Design review of the part built by this model. Coordinates are the model's own, in mm. Round coordinates to 2 decimals unless told otherwise and drop trailing zeros. Loops run counter-clockwise (first coordinate to the right, second up) from the corner with the lowest first, then second, coordinate; pieces in that order, holes last. Notation, with made-up numbers: (2.25, 9) - (48.25, 9) arc R21 ccw to (48.25, 27) - close; hole circle Ø5 at (-12.75, 34.5). An arc over 180 degrees is marked (long way). Return JSON: item names as keys, results as strings. Group by question number.
from build123d import *

# Parameters (mm, degrees)
SKETCH1_W           = 144.4
SKETCH1_H           = 144.4
BOSS_EXTRUDE1_DEPTH = 3
SKETCH2_W           = 20.628571
SKETCH2_H           = 3
SKETCH2_W_2         = 3
SKETCH2_H_2         = 19.771429
SKETCH2_H_3         = 19.83347722
SKETCH2_H_4         = 19.833479362
SKETCH2_H_5         = 19.771431142
CUT_EXTRUDE1_DEPTH  = 4
SKETCH3_R           = 1
CUT_EXTRUDE2_DEPTH  = 4
SKETCH4_R           = 4.8
CUT_EXTRUDE3_DEPTH  = 4


with BuildPart() as part:
    # Sketch1 → Boss-Extrude1 (new body)
    with BuildSketch(Plane.XY):
        Rectangle(SKETCH1_W, SKETCH1_H)
    extrude(amount=BOSS_EXTRUDE1_DEPTH)

    # Sketch2 → Cut-Extrude1 (cut, through all)
    with BuildSketch(Plane(origin=(0, 0, 0), x_dir=(-1, 0, 0), z_dir=(0, 0, -1))):
        with Locations((-41.257140929, 70.7)):
            Rectangle(SKETCH2_W, SKETCH2_H)
        with Locations((1.071e-06, 70.7)):
            Rectangle(SKETCH2_W, SKETCH2_H)
        with Locations((41.257143071, 70.7)):
            Rectangle(SKETCH2_W, SKETCH2_H)
        with Locations((70.7, 39.542856929)):
            Rectangle(SKETCH2_W_2, SKETCH2_H_2)
        with Locations((70.7, -1.071e-06)):
            Rectangle(SKETCH2_W_2, SKETCH2_H_2)
        with Locations((70.7, -39.573883181)):
            Rectangle(SKETCH2_W_2, SKETCH2_H_3)
        with Locations((41.257143071, -70.7)):
            Rectangle(SKETCH2_W, SKETCH2_H)
        with Locations((1.071e-06, -70.7)):
            Rectangle(SKETCH2_W, SKETCH2_H)
        with Locations((-41.257140929, -70.7)):
            Rectangle(SKETCH2_W, SKETCH2_H)
        with Locations((-70.7, -39.57388211)):
            Rectangle(SKETCH2_W_2, SKETCH2_H_4)
        with Locations((-70.7, 0)):
            Rectangle(SKETCH2_W_2, SKETCH2_H_5)
        with Locations((-70.7, 39.542858)):
            Rectangle(SKETCH2_W_2, SKETCH2_H_5)
    extrude(amount=-CUT_EXTRUDE1_DEPTH, mode=Mode.SUBTRACT)

    # Sketch3 → Cut-Extrude2 (cut, through all)
    with BuildSketch(Plane(origin=(0, 0, 0), x_dir=(-1, 0, 0), z_dir=(0, 0, -1))):
        with Locations((5, 0)):
            Circle(SKETCH3_R)
        with Locations((2.5, -4.330127019)):
            Circle(SKETCH3_R)
        with Locations((-2.5, -4.330127019)):
            Circle(SKETCH3_R)
        with Locations((-5, 0)):
            Circle(SKETCH3_R)
        with Locations((-2.5, 4.330127019)):
            Circle(SKETCH3_R)
        with Locations((2.5, 4.330127019)):
            Circle(SKETCH3_R)
        with Locations((10, 0)):
            Circle(SKETCH3_R)
        with Locations((8.660254038, -5)):
            Circle(SKETCH3_R)
        with Locations((5, -8.660254038)):
            Circle(SKETCH3_R)
        with Locations((0, -10)):
            Circle(SKETCH3_R)
        with Locations((-5, -8.660254038)):
            Circle(SKETCH3_R)
        with Locations((-8.660254038, -5)):
            Circle(SKETCH3_R)
        with Locations((-10, 0)):
            Circle(SKETCH3_R)
        with Locations((-8.660254038, 5)):
            Circle(SKETCH3_R)
        with Locations((-5, 8.660254038)):
            Circle(SKETCH3_R)
        with Locations((0, 10)):
            Circle(SKETCH3_R)
        with Locations((5, 8.660254038)):
            Circle(SKETCH3_R)
        with Locations((8.660254038, 5)):
            Circle(SKETCH3_R)
        with Locations((15, 0)):
            Circle(SKETCH3_R)
        with Locations((14.488887394, -3.882285677)):
            Circle(SKETCH3_R)
        with Locations((12.990381057, -7.5)):
            Circle(SKETCH3_R)
        with Locations((10.606601718, -10.606601718)):
            Circle(SKETCH3_R)
        with Locations((7.5, -12.990381057)):
            Circle(SKETCH3_R)
        with Locations((3.882285677, -14.488887394)):
            Circle(SKETCH3_R)
        with Locations((0, -15)):
            Circle(SKETCH3_R)
        with Locations((-3.882285677, -14.488887394)):
            Circle(SKETCH3_R)
        with Locations((-7.5, -12.990381057)):
            Circle(SKETCH3_R)
        with Locations((-10.606601718, -10.606601718)):
            Circle(SKETCH3_R)
        with Locations((-12.990381057, -7.5)):
            Circle(SKETCH3_R)
        with Locations((-14.488887394, -3.882285677)):
            Circle(SKETCH3_R)
        with Locations((-15, 0)):
            Circle(SKETCH3_R)
        with Locations((-14.488887394, 3.882285677)):
            Circle(SKETCH3_R)
        with Locations((-12.990381057, 7.5)):
            Circle(SKETCH3_R)
        with Locations((-10.606601718, 10.606601718)):
            Circle(SKETCH3_R)
        with Locations((-7.5, 12.990381057)):
            Circle(SKETCH3_R)
        with Locations((-3.882285677, 14.488887394)):
            Circle(SKETCH3_R)
        with Locations((0, 15)):
            Circle(SKETCH3_R)
        with Locations((3.882285677, 14.488887394)):
            Circle(SKETCH3_R)
        with Locations((7.5, 12.990381057)):
            Circle(SKETCH3_R)
        with Locations((10.606601718, 10.606601718)):
            Circle(SKETCH3_R)
        with Locations((12.990381057, 7.5)):
            Circle(SKETCH3_R)
        with Locations((14.488887394, 3.882285677)):
            Circle(SKETCH3_R)
    extrude(amount=-CUT_EXTRUDE2_DEPTH, mode=Mode.SUBTRACT)

    # Sketch4 → Cut-Extrude3 (cut, through all)
    with BuildSketch(Plane.XY.offset(3)):
        with Locations((0, 45)):
            Circle(SKETCH4_R)
        with Locations((45, 0)):
            Circle(SKETCH4_R)
        with Locations((0, -45)):
            Circle(SKETCH4_R)
        with Locations((-45, 0)):
            Circle(SKETCH4_R)
    extrude(amount=-CUT_EXTRUDE3_DEPTH, mode=Mode.SUBTRACT)


solid = part.part
Q1. Add section A-A, the plane x = -45. State the section outline as (y, z) points.
Q2. Draft analysis for pull direction Y (two halves, no side actions). For faces 1 (the flat face through (-1, 1, 0)), 2 (the cylindrical face through (49.58, 1.44, 1.52)), state which applies: pulls with the +Y half, pulls with the -Y half, needs draft (parallel to the pull), parting line crosses it, or undercut.
Q3. For line 1 (Y direction, x = 2, z = 2.6); line 2 (X direction, y = -9.5, z = 2.35); line 3 (X direction, y = 47, z = 0.25), list the stretches that pass through material, from the lowest coordinate up.
Q4. Add section C-C, the plane z = 1.2. Give the number of separate pieces and of enclosed holes in the cut face, plus the area to 3 significant figures.
Q5. Insertion check: pin 1 Ø0.9 at (x, z) = (41, 2) entering from -Y; pin 2 Ø1 at (x, z) = (-43.5, 2.5) entering from +Y. Each pin has a flat end and moves straight along its axis. Give the tip position at first contact, or say it passes through.
Evaluation:
{
 "1": {"outline": "(-69.2, 0) - (-4.8, 0) - (-4.8, 3) - (-69.2, 3) - close; (4.8, 0) - (69.2, 0) - (69.2, 3) - (4.8, 3) - close"},
 "2": {"face 1": "needs draft", "face 2": "undercut"},
 "3": {"line 1": "-69.2 to -49.36, -40.64 to -5.2, -3.46 to 3.46, 5.2 to 40.64, 49.36 to 69.2", "line 2": "-69.2 to -5.54, -4.46 to -0.87, 0.87 to 4.46, 5.54 to 69.2", "line 3": "-69.2 to -4.36, 4.36 to 69.2"},
 "4": {"separate pieces": "1", "enclosed holes": "46", "area": "19,700 mm²"},
 "5": {"pin 1": "y = -69.2", "pin 2": "y = 69.2"}
}
